```python
from build123d import *

# Parameters (mm, degrees)
BOSS_EXTRUDE1_DEPTH = 3.175
CUT_EXTRUDE1_DEPTH  = 84.508560046


with BuildPart() as part:
    # Sketch1 → Boss-Extrude1 (new body)
    with BuildSketch(Plane.XY):
        Polygon((-61.976, 0), (0, 55.88), (0, 0), (-11.43, 0), (-11.43, -3.175), (-49.784, -3.175), (-49.784, 0), align=None)
    extrude(amount=BOSS_EXTRUDE1_DEPTH)

    # Sketch2 → Cut-Extrude1 (cut, through all)
    with BuildSketch(Plane.XY.offset(3.175)):
        Polygon((-3.58, 11), (-3.58, 8.45), (-2.28, 8.45), (-2.28, 6.55), (-3.58, 6.55), (-3.58, 0), (-6.58, 0), (-6.58, 6.55), (-7.88, 6.55), (-7.88, 8.45), (-6.58, 8.45), (-6.58, 11), align=None)
    extrude(amount=-CUT_EXTRUDE1_DEPTH, mode=Mode.SUBTRACT)


solid = part.part
```
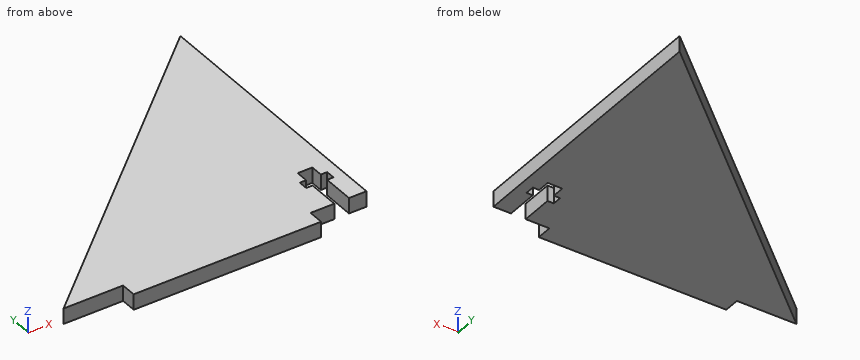
Here's how the part is built. I have some questions about the finished solid (model axes, mm). Give positions to 0.01 mm unless a question says otherwise; leave off trailing zeros. Write each loop counter-clockwise with the first axis right and the second up, starting at its lowest first coordinate (ties: lowest second). Pieces come first, ordered by that corner, then holes. Notation, with made-up numbers: M -33.75,55 L 16.25,55 A27 cw 16.25,73 Z; hole C 71.25,-12.75 d10. An arc over 180 degrees is marked long. Put each result on its own line as item: value. Start each with the question number.
Item 1: If we section it at C-C, the plane x = -16: Write out the boundary of the cut face in (y, z) (3 decimals), then the cut area to 3 significant figures.
Item 2: If we section it at A-A, the plane z = 1.4: Write out the boundary of the cut face in (x, y) (3 decimals), then the cut area to 3 significant figures.
Item 3: Will these pins go through, and if not, where does the flat tip stop? pin 1 (1.4 mm diameter, centred on x = -7, z = 1, fed in from +Y); pin 2 (1.6 mm diameter, centred on x = -2, z = 1, fed in from -Y); pin 3 (1 mm diameter, centred on y = -1, z = 2, fed in from +X).
Item 4: If we section it at B-B, the plane y = 34: Write out the boundary of the cut face in (x, z) (3 decimals), then the cut area to 3 significant figures.
Item 5: I need wall thicknesses on L1, parallel to Y at x = -2.5, z = 1.7; L2, parallel to X at y = 5.5, z = 1.8; L3, parallel to X at y = 4.5, z = 1.15. Which ranges of each line are inside material? Lowest first, please. Write a range as from..to.
Values:
1. outline: M -3.175,0 L 41.454,0 L 41.454,3.175 L -3.175,3.175 Z
1. area: 142 mm²
2. outline: M -61.976,0 L -49.784,0 L -49.784,-3.175 L -11.43,-3.175 L -11.43,0 L -6.58,0 L -6.58,6.55 L -7.88,6.55 L -7.88,8.45 L -6.58,8.45 L -6.58,11 L -3.58,11 L -3.58,8.45 L -2.28,8.45 L -2.28,6.55 L -3.58,6.55 L -3.58,0 L 0,0 L 0,55.88 Z
2. area: 1,820 mm²
3. pin 1: y = 50.2
3. pin 2: y = 0
3. pin 3: x = -11.43
4. outline: M -24.267,0 L 0,0 L 0,3.175 L -24.267,3.175 Z
4. area: 77.0 mm²
5. L1: 0..6.55, 8.45..53.63
5. L2: -55.88..-6.58, -3.58..0
5. L3: -56.99..-6.58, -3.58..0
